Job drawing, mm, ordinate dimensions from the low corner. One solid piece. A direction names the side the tool comes from. Coordinates: 2 decimals unless noted, no trailing zeros. Loops run counter-clockwise (first coordinate to the right, second up) from the corner with the lowest first, then second, coordinate; pieces in that order, holes last. Notation, with made-up numbers: M 31,-0.75 L 41,-0.75 A6 cw 41,6.25 Z; hole C 71.25,66 d6. An arc over 180 degrees is marked long. Answer as a JSON object with one key per item and string values. Group by question number.
1. Drill centre lines: L1, parallel to X at y = 36, z = 21.5 (1 decimal); L2, parallel to Y at x = 27, z = 16.5 (1 decimal); L3, parallel to Z at x = 13.5, y = 24.5. Where is each one in solid material? Low to high.
2. Drop flat-ended pins along their axis: pin 1 Ø4 at (x, z) = (21, 7.5) entering from +Y; pin 2 Ø12.5 at (x, y) = (11, 34) entering from -Z; pin 3 Ø6.5 at (x, z) = (17.5, 4) entering from -Y. Give the stop position or say it passes through.
3. 3-axis set-ups, long thin cutter, end or side, ignore diameter. For the marked faces 1, 2 and 3: which of +Z, -Z, +X, -X, +Y, -Y reach the whole face in a straight line?
4. Saw through at B-B on z = 18. Write the cut outline in (x, y) (1 decimal).
5. Saw through at D-D on x = 32. Write the cut outline in (y, z) (1 decimal), then the cut area to 3 significant figures.
6. Saw through at A-A on x = 19. Write the cut outline in (y, z) (1 decimal).
7. Saw through at C-C on y = 26. Write the cut outline in (x, z) (1 decimal).
8. Mould opens along X. For the marked faces 4, 5, 6 and 7 say: released by +X, released by -X, zero draft, split by the parting line, or undercut.
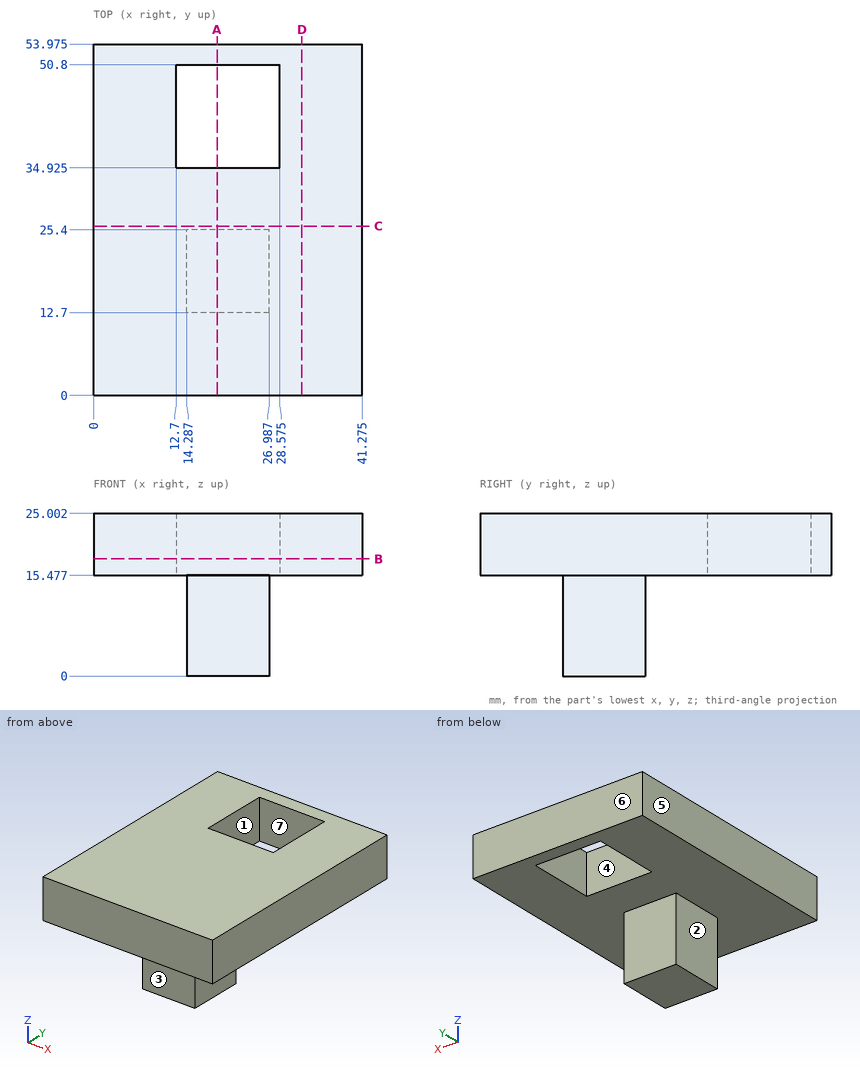
Outcome:
{
 "1": {"L1": "x = 0 to 12.7, 28.6 to 41.3", "L2": "y = 0 to 34.9, 50.8 to 54", "L3": "z = 15.48 to 25"},
 "2": {"pin 1": "stops at y = 25.4", "pin 2": "stops at z = 15.48", "pin 3": "stops at y = 12.7"},
 "3": {"face 1": "+Z, -Z", "face 2": "-Z, -X, +Y, -Y", "face 3": "-Z, +X, -X, -Y"},
 "4": {"outline": "M 0,0 L 41.3,0 L 41.3,54 L 0,54 Z; hole M 12.7,34.9 L 28.6,34.9 L 28.6,50.8 L 12.7,50.8 Z"},
 "5": {"outline": "M 0,15.5 L 54,15.5 L 54,25 L 0,25 Z", "area": "514 mm²"},
 "6": {"outline": "M 0,15.5 L 12.7,15.5 L 12.7,0 L 25.4,0 L 25.4,15.5 L 34.9,15.5 L 34.9,25 L 0,25 Z; M 50.8,15.5 L 54,15.5 L 54,25 L 50.8,25 Z"},
 "7": {"outline": "M 0,15.5 L 41.3,15.5 L 41.3,25 L 0,25 Z"},
 "8": {"face 4": "undercut", "face 5": "released by -X", "face 6": "zero draft", "face 7": "undercut"}
}
